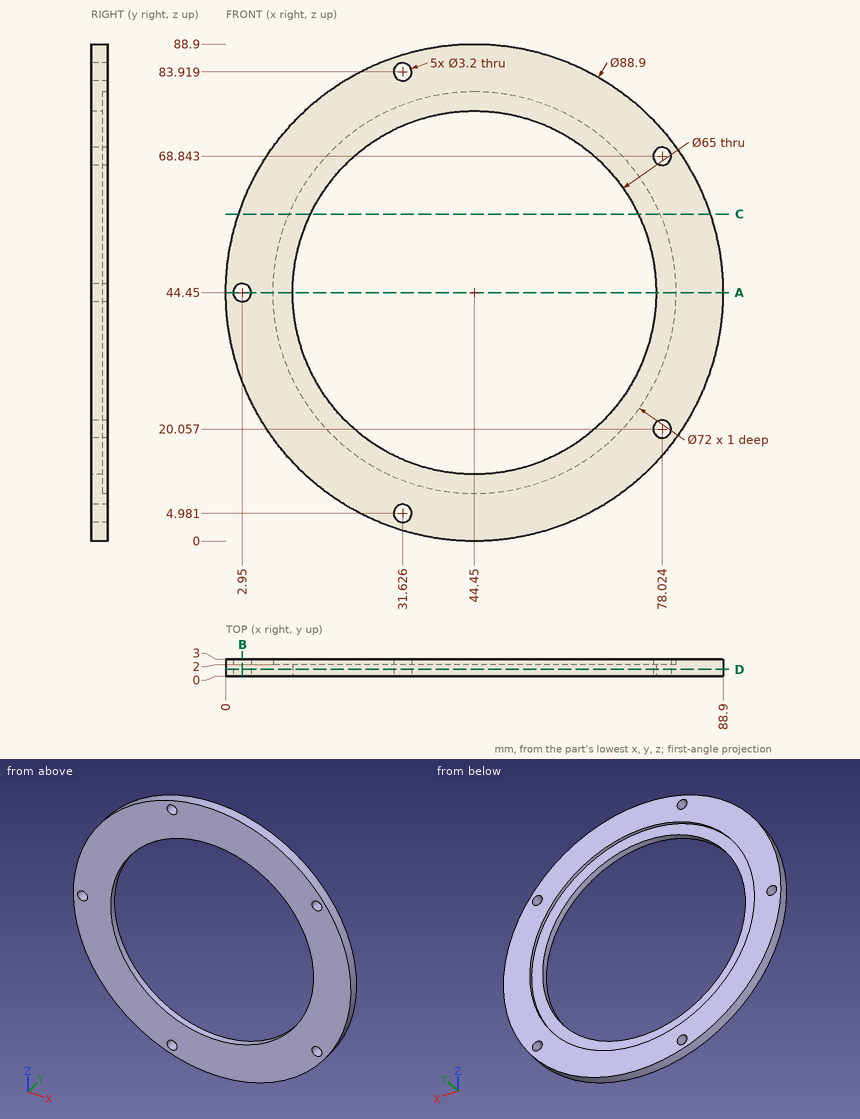
For this review, use the dimensioned drawing (mm, ordinates from the lowest corner) and the shaded views. Give positions to 0.01 mm unless a question says otherwise; leave off trailing zeros. Order: outer loops, then holes, each group sorted by start corner. A loop starts at its lowest first (then second) coordinate and runs counter-clockwise, first axis right, second up.
1) Take a section at D-D (y = 1.2). Give the boundary of the cut face in (x, z), then the cut area to 3 significant figures.
2) Take a section at A-A (z = 44.45). Give the boundary of the cut face in (x, y), then the cut area to 3 significant figures.
3) Wall thickness on line 1 (X direction, y = 2.3, z = 44.45); line 2 (Y direction, x = 65, z = 71); line 3 (Z direction, x = 70, y = 2.3): over which ranges is each line inside the solid? List them lowest first.
4) Insertion check: pin 1 (4 mm diameter, centred on x = 2.95, z = 44.45, fed in from -Y); pin 2 (1.5 mm diameter, centred on x = 32.5, y = 1, fed in from -Z); pin 3 (1 mm diameter, centred on y = 0.5, z = 70, fed in from +X). Each pin has a flat end and moves straight along its axis. Give the tip position at first contact, or say it passes through.
5) Take a section at C-C (z = 58.5). Give the boundary of the cut face in (x, y) (1 decimal).
6) Take a section at B-B (x = 2.95). Give the boundary of the cut face in (y, z).
Derived:
1. outline: circle Ø88.9 at (44.45, 44.45); hole circle Ø3.2 at (2.95, 44.45); hole circle Ø65 at (44.45, 44.45); hole circle Ø3.2 at (31.63, 4.98); hole circle Ø3.2 at (31.63, 83.92); hole circle Ø3.2 at (78.02, 20.06); hole circle Ø3.2 at (78.02, 68.84)
1. area: 2,850 mm2
2. outline: (0, 0) - (1.35, 0) - (1.35, 3) - (0, 3) - close; (4.55, 0) - (11.95, 0) - (11.95, 2) - (8.45, 2) - (8.45, 3) - (4.55, 3) - close; (76.95, 0) - (88.9, 0) - (88.9, 3) - (80.45, 3) - (80.45, 2) - (76.95, 2) - close
2. area: 55.1 mm2
3. line 1: x = 0 to 1.35, 4.55 to 8.45, 80.45 to 88.9
3. line 2: y = 0 to 2
3. line 3: z = 8.08 to 19.09, 69.81 to 80.82
4. pin 1: stops at y = 0
4. pin 2: stops at z = 1.43
4. pin 3: stops at x = 81.17
5. outline: (2.3, 0) - (15.1, 0) - (15.1, 2) - (11.3, 2) - (11.3, 3) - (2.3, 3) - close; (73.8, 0) - (86.6, 0) - (86.6, 3) - (77.6, 3) - (77.6, 2) - (73.8, 2) - close
6. outline: (0, 28.53) - (3, 28.53) - (3, 42.85) - (0, 42.85) - close; (0, 46.05) - (3, 46.05) - (3, 60.37) - (0, 60.37) - close
